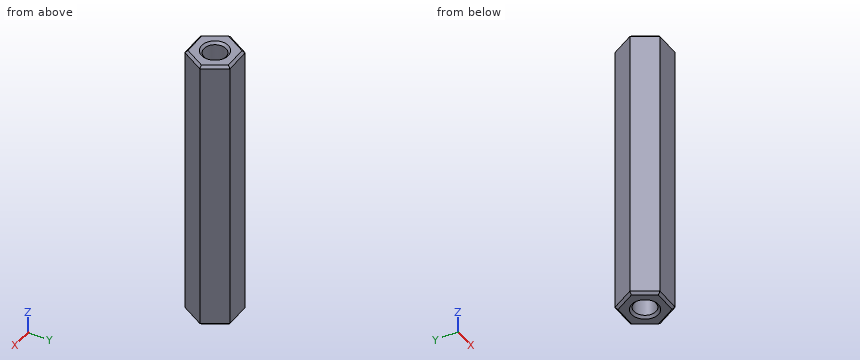
Autodesk Inventor part; units mm, degrees
ref_plane "YZ Plane" through (0, 0, 0) normal (1, 0, 0) x (0, 1, 0)
ref_plane "XZ Plane" through (0, 0, 0) normal (0, 1, 0) x (-1, 0, 0)
ref_plane "XY Plane" through (0, 0, 0) normal (0, 0, 1) x (1, 0, 0)
sketch "Sketch1" plane through (0, 0, 0) normal (0, 0, 1) x (1, 0, 0)
  line L0 (1.3712, 2.375) -> (2.7424, 0)
  line L1 (2.7424, 0) -> (1.3712, -2.375)
  line L2 (1.3712, -2.375) -> (-1.3712, -2.375)
  line L3 (-1.3712, -2.375) -> (-2.7424, 0)
  line L4 (-2.7424, 0) -> (-1.3712, 2.375)
  line L5 (-1.3712, 2.375) -> (1.3712, 2.375)
  circle A0 centre (0, 0) radius 1.175
  dimension "d0" = 4.75
  dimension "d1" = 2.35
extrude "Extrusion1" add sketch "Sketch1" along normal blind 30
thread "Thread1"
chamfer "Chamfer1" distance 0.25 angle 45 14 edges at (0, 2.375, 30) (-2.0568, 1.1875, 30) (-2.0568, -1.1875, 30) (2.0568, -1.1875, 30) (2.0568, 1.1875, 30) (2.0568, 1.1875, 0) (0, 2.375, 0) (-2.0568, 1.1875, 0) (-2.0568, -1.1875, 0) (-1.175, 0, 0) (0, -2.375, 0) (2.0568, -1.1875, 0) (-1.175, 0, 30) (0, -2.375, 30)
properties part number "Part3_Poste largo de latón"
Verification items for the finished model (mm, model axes). Give positions to 0.01 mm unless a question says otherwise; leave off trailing zeros. Loops run counter-clockwise (first coordinate to the right, second up) from the corner with the lowest first, then second, coordinate; pieces in that order, holes last. Notation, with made-up numbers: (74, 54.5) - (80, 54.5) arc R20 cw to (80, 71.5) - close; hole circle Ø4 at (-19.75, 27). An arc over 180 degrees is marked (long way). Write item = value, one per line. Start each with the question number.
Q1. Thickness scan on line 1 (Y direction, x = 0, z = 20.25) (3 decimals); line 2 (X direction, y = -1.05, z = 28); line 3 (Y direction, x = 0.7, z = 8) (3 decimals). Record the ranges inside material, lowest first.
Q2. Cross-section at C-C, the plane x = -2.2. Enter the section's corners in (y, z), and give its area (3 significant figures).
Q3. Cross-section at B-B, the plane x = 0. Enter the section's corners in (y, z) (3 decimals).
Q4. Cross-section at A-A, the plane z = 26. Enter the section's corners in (x, y) (3 decimals), and give its area (3 significant figures).
Q5. Depth check by flat-ended pin: P1, Ø1.5, axis at x = 1.5, y = 1, coming from the -Z side. Enter the tip coordinate at first touch or a pass-through.
Q6. Cross-section at D-D, the plane x = 1.8. Enter the section's corners in (y, z).
Answer key:
q1.line_1 = -2.375 to -1.175, 1.175 to 2.375
q1.line_2 = -2.14 to -0.53, 0.53 to 2.14
q1.line_3 = -2.375 to -0.944, 0.944 to 2.375
q2.outline = (-0.94, 0.25) - (-0.44, 0) - (0.44, 0) - (0.94, 0.25) - (0.94, 29.75) - (0.44, 30) - (-0.44, 30) - (-0.94, 29.75) - close
q2.area = 56.1 mm^2
q3.outline = (-2.375, 0.25) - (-2.125, 0) - (-1.425, 0) - (-1.175, 0.25) - (-1.175, 29.75) - (-1.425, 30) - (-2.125, 30) - (-2.375, 29.75) - close; (1.175, 0.25) - (1.425, 0) - (2.125, 0) - (2.375, 0.25) - (2.375, 29.75) - (2.125, 30) - (1.425, 30) - (1.175, 29.75) - close
q4.outline = (-2.742, 0) - (-1.371, -2.375) - (1.371, -2.375) - (2.742, 0) - (1.371, 2.375) - (-1.371, 2.375) - close; hole circle Ø2.35 at (0, 0)
q4.area = 15.2 mm^2
q5.P1 = 0
q6.outline = (-1.63, 0.25) - (-1.13, 0) - (1.13, 0) - (1.63, 0.25) - (1.63, 29.75) - (1.13, 30) - (-1.13, 30) - (-1.63, 29.75) - close
